Answer from the drawing. Dimensions are ordinates in mm from the lowest x, y and z of the part. A direction names the side the tool comes from. Coordinates: 2 decimals unless noted, no trailing zeros. Write each loop counter-clockwise with the first axis right and the second up, starting at its lowest first coordinate (ties: lowest second). Pieces come first, ordered by that corner, then holes. Notation, with made-up numbers: (-28, 6.25) -> (-21, 6.25) arc R26 ccw to (-21, 21.25) -> close; hole circle Ø2 at (78.25, 36.25). An arc over 180 degrees is marked (long way). One line per item, written item: value. Start each with the question number.
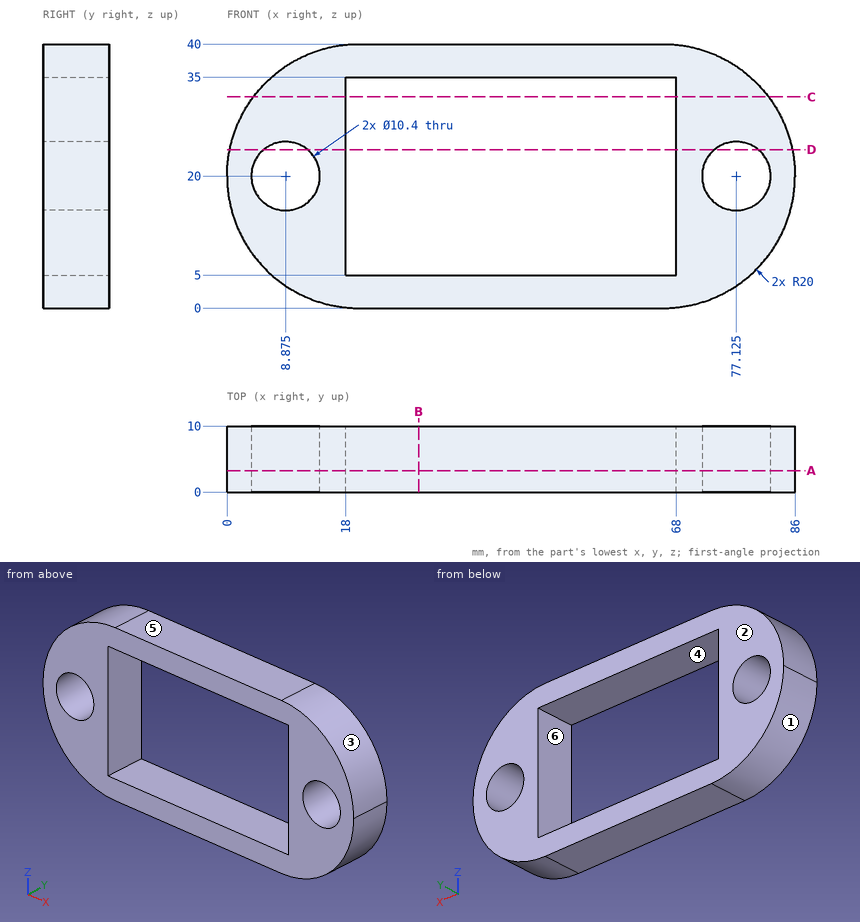
1. A cutting plane is placed at C-C on z = 32. Give the vertices of the cut face in (x, y).
2. For a pull along Z with two mould halves and no side action, classify the marked faces 1, 2, 3 and 4 as +Z half, -Z half, draft (parallel to the pull), parting line (faces both ways), or undercut.
3. Given pin 1 (3 mm diameter, centred on y = 5, z = 22, fed in from +X); pin 2 (1 mm diameter, centred on y = 8, z = 17.5, fed in from +X); pin 3 (4 mm diameter, centred on x = 13.5, y = 2, fed in from +Z), each flat-ended and moving along its own axis, determine where each tip first touches the part or whether it passes through.
4. Find the intervals of material crossed by probe 1 along Z at (x, y) = (36, 1.5); probe 2 along X at (y, z) = (2.5, 15.5); probe 3 along X at (y, z) = (8.75, 23), in increasing order. Write a range as from..to.
5. A cutting plane is placed at D-D on z = 24. Give the vertices of the cut face in (x, y), then the cut area to 3 significant figures.
6. A tool of negligible diameter and unlimited length cuts with its end or side. For the marked faces 5 and 6, from which of +Z, -Z, +X, -X, +Y, -Y can it reach the whole face along a straight path? Write none if from no direction.
7. A cutting plane is placed at B-B on x = 29. Give the vertices of the cut face in (y, z).
8. A cutting plane is placed at A-A on y = 3.25. Count the separate pieces of the cut face and the enclosed holes in it, then the cut area to 3 significant figures.
Derived:
1. outline: (4, 0) -> (18, 0) -> (18, 10) -> (4, 10) -> close; (68, 0) -> (82, 0) -> (82, 10) -> (68, 10) -> close
2. face 1: -Z half
2. face 2: draft
2. face 3: +Z half
2. face 4: undercut
3. pin 1: stops at x = 85.99
3. pin 2: stops at x = 85.9
3. pin 3: stops at z = 39.49
4. probe 1: z = 0..5, 35..40
4. probe 2: x = 0.51..6.27, 11.48..18, 68..74.52, 79.73..85.49
4. probe 3: x = 0.23..4.63, 13.12..18, 68..72.88, 81.37..85.77
5. outline: (0.4, 0) -> (5.55, 0) -> (5.55, 10) -> (0.4, 10) -> close; (12.2, 0) -> (18, 0) -> (18, 10) -> (12.2, 10) -> close; (68, 0) -> (73.8, 0) -> (73.8, 10) -> (68, 10) -> close; (80.45, 0) -> (85.6, 0) -> (85.6, 10) -> (80.45, 10) -> close
5. area: 219 mm2
6. face 5: +Z, +X, -X, +Y, -Y
6. face 6: +Y, -Y
7. outline: (0, 0) -> (10, 0) -> (10, 5) -> (0, 5) -> close; (0, 35) -> (10, 35) -> (10, 40) -> (0, 40) -> close
8. separate pieces: 1
8. enclosed holes: 3
8. area: 1,430 mm2
